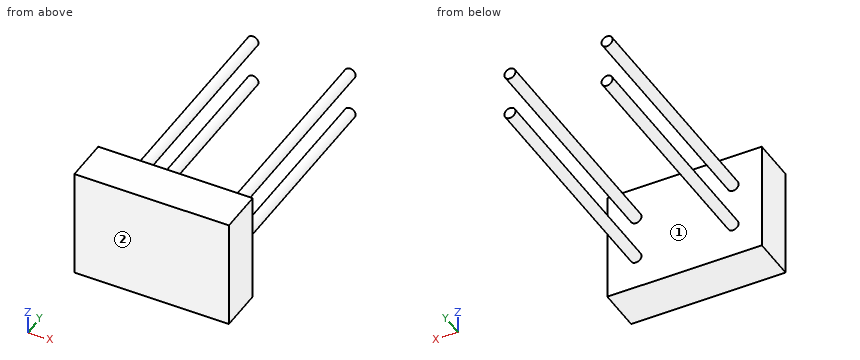
from build123d import *

# Parameters (mm, degrees)
SKETCH1_W           = 350
SKETCH1_H           = 250
BOSS_EXTRUDE1_DEPTH = 100
SKETCH3_R           = 12.5
BOSS_EXTRUDE2_DEPTH = 530


with BuildPart() as part:
    # Sketch1 → Boss-Extrude1 (new body)
    with BuildSketch(Plane(origin=(0, 0, 0), x_dir=(1, 0, 0), z_dir=(0, 1, 0))):
        Rectangle(SKETCH1_W, SKETCH1_H)
    extrude(amount=BOSS_EXTRUDE1_DEPTH)

    # Sketch3 → Boss-Extrude2 (add)
    with BuildSketch(Plane(origin=(0, 100, 0), x_dir=(1, 0, 0), z_dir=(0, 1, 0))):
        with Locations((-110, 50)):
            Circle(SKETCH3_R)
        with Locations((110, 50)):
            Circle(SKETCH3_R)
        with Locations((110, -50)):
            Circle(SKETCH3_R)
        with Locations((-110, -50)):
            Circle(SKETCH3_R)
    extrude(amount=BOSS_EXTRUDE2_DEPTH)


solid = part.part
The listing builds one solid part. Answer for the finished solid, in the listing's coordinates (mm). Face numbers are marked on the shaded views. A direction names the side the tool comes from. Give positions to 0.01 mm unless a question says otherwise; leave off trailing zeros. Write each loop counter-clockwise with the first axis right and the second up, starting at its lowest first coordinate (ties: lowest second). Pieces come first, ordered by that corner, then holes. Notation, with made-up numbers: (55, -25.75) - (86, -25.75) arc R18 cw to (86, -13.75) - close; hole circle Ø6 at (-24.75, 89). An arc over 180 degrees is marked (long way). Use a Markdown table: item, result.
1. A tool of negligible diameter and unlimited length cuts with its end or side. For the marked faces 1 and 2, from which of +Z, -Z, +X, -X, +Y, -Y can it reach the whole face along a straight path? Write none if from no direction.
Values follow:
| item | result |
|---|---|
| face 1 | +Y |
| face 2 | +Z, -Z, +X, -X, -Y |
2. Section D-D on z = -94 is taken. Write down the section's boundary in (x, y), plus the area to 3 significant figures.
Values follow:
| item | result |
|---|---|
| outline | (-175, 0) - (175, 0) - (175, 100) - (-175, 100) - close |
| area | 35,000 mm² |
3. Section C-C on y = 458.5 is taken. Write down the section's boundary in (x, z), plus the area to 3 significant figures.
Values follow:
| item | result |
|---|---|
| outline | circle Ø25 at (-110, -50); circle Ø25 at (-110, 50); circle Ø25 at (110, -50); circle Ø25 at (110, 50) |
| area | 1,960 mm² |
4. Section A-A on z = -50 is taken. Write down the section's boundary in (x, y), plus the area to 3 significant figures.
Values follow:
| item | result |
|---|---|
| outline | (-175, 0) - (175, 0) - (175, 100) - (122.5, 100) - (122.5, 630) - (97.5, 630) - (97.5, 100) - (-97.5, 100) - (-97.5, 630) - (-122.5, 630) - (-122.5, 100) - (-175, 100) - close |
| area | 61,500 mm² |
5. Section B-B on x = -106.5 is taken. Write down the section's boundary in (y, z), plus the area to 3 significant figures.
Values follow:
| item | result |
|---|---|
| outline | (0, -125) - (100, -125) - (100, -62) - (630, -62) - (630, -38) - (100, -38) - (100, 38) - (630, 38) - (630, 62) - (100, 62) - (100, 125) - (0, 125) - close |
| area | 50,400 mm² |
6. Find the intervals of material crossed by probe 1 along X at (y, z) = (588.5, 49); probe 2 along Y at (x, z) = (-102.5, -73.5); probe 3 along Z at (x, y) = (113, 193.5), in increasing order. Write a range as from..to.
Values follow:
| item | result |
|---|---|
| probe 1 | x = -122.46..-97.54, 97.54..122.46 |
| probe 2 | y = 0..100 |
| probe 3 | z = -62.13..-37.87, 37.87..62.13 |
7. Each of these flat-tipped pins is pushed along its axis until it touches: P1, Ø8, axis at y = 451, z = -41, coming from the +X side; P2, Ø10, axis at y = 359, z = 36.5, coming from the +X side; P3, Ø4, axis at x = 8.5, z = -49, coming from the -Y side; P4, Ø5, axis at x = 108.5, y = 407, coming from the +Z side. Where does it stop, or does it pass through?
Values follow:
| item | result |
|---|---|
| P1 | stops at x = 121.46 |
| P2 | stops at x = 119.17 |
| P3 | stops at y = 0 |
| P4 | stops at z = 62.5 |
